Input: part model. Units: mm. Frame: model coordinates. A direction names the side the tool comes from. Round coordinates to 2 decimals unless told otherwise and drop trailing zeros. Order: outer loops, then holes, each group sorted by start corner. A loop starts at its lowest first (then second) coordinate and runs counter-clockwise, first axis right, second up. Notation, with made-up numbers: (-7.75, 39) -> (13.25, 39) arc R23 cw to (13.25, 69) -> close; hole circle Ø4 at (65, 22.5). An arc over 180 degrees is marked (long way). Use a Markdown table: item, result.
from build123d import *

# Parameters (mm, degrees)
SKETCH1_R           = 3.175
BOSS_EXTRUDE1_DEPTH = 6.35
FILLET1_R           = 6.35
FILLET2_R           = 12.7
SKETCH2_R           = 4.9625
CUT_EXTRUDE1_DEPTH  = 4.7625
SKETCH5_R           = 1.778
CUT_EXTRUDE3_DEPTH  = 66.013999766
CUT_EXTRUDE15_DEPTH = 66.013999766
SKETCH11_R          = 3.1702
CUT_EXTRUDE16_DEPTH = 3.175
BOSS_EXTRUDE2_START = -6.35
BOSS_EXTRUDE2_DEPTH = 6.35
SKETCH12_W          = 25.4
SKETCH12_H          = 12.7
CUT_EXTRUDE17_DEPTH = 63.747431864
FILLET14_R          = 3.175
CHAMFER4_SIZE       = 0.4
FILLET16_R          = 3.175
FILLET17_R          = 3.175
SKETCH16_R          = 3.375
BOSS_EXTRUDE4_DEPTH = 6.35
SKETCH17_R          = 3.375
CUT_EXTRUDE19_DEPTH = 69.950310788
FILLET19_R          = 6.35
FILLET20_R          = 9.525


with BuildPart() as part:
    # Sketch1 → Boss-Extrude1 (new body)
    with BuildSketch(Plane.XY):
        with BuildLine():
            Line((-19.735202783, 15.926469991), (-23.822191281, 21.144118554))
            ThreePointArc((-23.822191281, 21.144118554), (-23.438788835, 29.420896018), (-15.197028879, 30.272621002))
            Line((-15.197028879, 30.272621002), (-1.135121582, 20.490721215))
            Line((-1.135121582, 20.490721215), (26.988693011, 20.490721215))
            Line((26.988693011, 20.490721215), (42.638100307, 30.272621002))
            ThreePointArc((42.638100307, 30.272621002), (50.879860264, 29.420896018), (51.263262709, 21.144118554))
            Line((51.263262709, 21.144118554), (47.176274212, 15.926469991))
            Line((47.176274212, 15.926469991), (47.176274212, 5.491172866))
            Line((47.176274212, 5.491172866), (51.263262709, 0.273524304))
            ThreePointArc((51.263262709, 0.273524304), (52.267035248, -1.571068231), (52.614285714, -3.642178571))
            Line((52.614285714, -3.642178571), (52.614285714, -37.65945571))
            Line((52.614285714, -37.65945571), (-25.173214286, -37.65945571))
            Line((-25.173214286, -37.65945571), (-25.173214286, -3.642178571))
            ThreePointArc((-25.173214286, -3.642178571), (-24.825963819, -1.571068231), (-23.822191281, 0.273524304))
            Line((-23.822191281, 0.273524304), (-19.735202783, 5.491172866))
            Line((-19.735202783, 5.491172866), (-19.735202783, 15.926469991))
        make_face()
        with Locations((-18.823214286, 25.059821429)):
            Circle(SKETCH1_R, mode=Mode.SUBTRACT)
        with Locations((46.264285714, 25.059821429)):
            Circle(SKETCH1_R, mode=Mode.SUBTRACT)
        with Locations((46.264285714, -3.642178571)):
            Circle(SKETCH1_R, mode=Mode.SUBTRACT)
        with Locations((-18.823214286, -3.642178571)):
            Circle(SKETCH1_R, mode=Mode.SUBTRACT)
    extrude(amount=BOSS_EXTRUDE1_DEPTH)

    # Fillet1
    fillet1_edges = [part.edges().sort_by_distance(p)[0] for p in [
        (47.176274212, 15.926469991, 3.175),
        (47.176274212, 5.491172866, 3.175),
        (-19.735202783, 5.491172866, 3.175),
        (-19.735202783, 15.926469991, 3.175),
    ]]
    fillet(fillet1_edges, radius=FILLET1_R)

    # Fillet2
    fillet2_edges = [part.edges().sort_by_distance(p)[0] for p in [
        (-1.135121582, 20.490721215, 3.175),
        (26.988693011, 20.490721215, 3.175),
    ]]
    fillet(fillet2_edges, radius=FILLET2_R)

    # Sketch2 → Cut-Extrude1 (cut)
    with BuildSketch(Plane.XY.offset(6.35)):
        with Locations((-18.823214286, 25.059821429)):
            Circle(SKETCH2_R)
        with Locations((-18.823214286, -3.642178571)):
            Circle(SKETCH2_R)
        with Locations((46.264285714, -3.642178571)):
            Circle(SKETCH2_R)
        with Locations((46.264285714, 25.059821429)):
            Circle(SKETCH2_R)
    extrude(amount=-CUT_EXTRUDE1_DEPTH, mode=Mode.SUBTRACT)

    # Sketch5 → Cut-Extrude3 (cut, through all)
    with BuildSketch(Plane(origin=(0, 0, 0), x_dir=(-1, 0, 0), z_dir=(0, 0, -1))):
        with Locations((21.423664788, -18.813799362)):
            Circle(SKETCH5_R)
        with Locations((21.423664788, -28.813754296)):
            Circle(SKETCH5_R)
        with Locations(Location((-26.876213212, -28.813754296, 0), (0, 0, 180))):
            Circle(SKETCH5_R)
        with Locations(Location((-26.876213212, -18.813799362, 0), (0, 0, 180))):
            Circle(SKETCH5_R)
    extrude(amount=-CUT_EXTRUDE3_DEPTH, mode=Mode.SUBTRACT)

    # Sketch6 → Cut-Extrude15 (cut, through all)
    with BuildSketch(Plane.XY.offset(6.35)):
        Polygon((-18.228725788, -33.59545571), (-25.173214286, -33.59545571), (-25.173214286, -37.65945571), (-17.553214286, -37.65945571), (-8.028214286, -37.65945571), (33.881785714, -37.65945571), (43.406785714, -37.65945571), (51.026785714, -37.65945571), (52.614285714, -37.65945571), (52.614285714, -4.530802681), (52.3703532, -5.385290691), (44.317137236, -33.59545571), (23.681274212, -33.59545571), (23.681274212, -13.78345571), (-18.228725788, -13.78345571), align=None)
    extrude(amount=-CUT_EXTRUDE15_DEPTH, mode=Mode.SUBTRACT)

    # Sketch11 → Cut-Extrude16 (cut)
    with BuildSketch(Plane.XY.offset(6.35)):
        with Locations((-21.423664788, -18.813799362)):
            Circle(SKETCH11_R)
        with Locations((-21.423664788, -28.813754296)):
            Circle(SKETCH11_R)
        with Locations((26.876213212, -28.813754296)):
            Circle(SKETCH11_R)
        with Locations((26.876213212, -18.813799362)):
            Circle(SKETCH11_R)
    extrude(amount=-CUT_EXTRUDE16_DEPTH, mode=Mode.SUBTRACT)

    # Sketch13 → Boss-Extrude2 (add)
    with BuildSketch(Plane.XY.offset(6.35).offset(BOSS_EXTRUDE2_START)):
        with BuildLine():
            Line((-30.928725788, -33.59545571), (-25.173214286, -33.59545571))
            Line((-25.173214286, -33.59545571), (-25.173214286, -3.642178571))
            ThreePointArc((-25.173214286, -3.642178571), (-24.825963819, -1.571068231), (-23.822191281, 0.273524304))
            Line((-23.822191281, 0.273524304), (-23.804629036, 0.295945121))
            Line((-23.804629036, 0.295945121), (-30.928725788, -8.632865637))
            Line((-30.928725788, -8.632865637), (-30.928725788, -33.59545571))
        make_face()
    extrude(amount=BOSS_EXTRUDE2_DEPTH)

    # Sketch12 → Cut-Extrude17 (cut, through all)
    with BuildSketch(Plane.XY.offset(6.35)):
        with Locations((12.7, 4.358821429)):
            Rectangle(SKETCH12_W, SKETCH12_H)
    extrude(amount=-CUT_EXTRUDE17_DEPTH, mode=Mode.SUBTRACT)

    # Fillet14
    fillet14_edges = [part.edges().sort_by_distance(p)[0] for p in [
        (0, -1.991178571, 3.175),
        (0, 10.708821429, 3.175),
        (25.4, 10.708821429, 3.175),
        (25.4, -1.991178571, 3.175),
    ]]
    fillet(fillet14_edges, radius=FILLET14_R)

    # Chamfer4
    chamfer4_edges = [part.edges().sort_by_distance(p)[0] for p in [
        (12.7, 10.708821429, 6.35),
        (12.7, 10.708821429, 0),
        (25.4, 4.358821429, 6.35),
        (25.4, 4.358821429, 0),
        (0, 4.358821429, 6.35),
        (0, 4.358821429, 0),
        (12.7, -1.991178571, 6.35),
        (12.7, -1.991178571, 0),
        (24.47006403, 9.778885459, 6.35),
        (24.47006403, 9.778885459, 0),
        (0.92993597, 9.778885459, 6.35),
        (0.92993597, 9.778885459, 0),
        (0.92993597, -1.061242602, 6.35),
        (0.92993597, -1.061242602, 0),
        (24.47006403, -1.061242602, 6.35),
        (24.47006403, -1.061242602, 0),
    ]]
    chamfer(chamfer4_edges, length=CHAMFER4_SIZE)

    # Fillet16
    fillet16_edges = [part.edges().sort_by_distance(p)[0] for p in [
        (-30.928725788, -33.59545571, 3.175),
        (-30.928725788, -8.632865637, 3.175),
    ]]
    fillet(fillet16_edges, radius=FILLET16_R)

    # Fillet17
    fillet17_edges = [part.edges().sort_by_distance(p)[0] for p in [
        (44.317137236, -33.59545571, 3.175),
    ]]
    fillet(fillet17_edges, radius=FILLET17_R)

    # Sketch16 → Boss-Extrude4 (add)
    # profile 1 of 2: a face of its own
    with BuildSketch(Plane.XY.offset(6.35)):
        with BuildLine():
            Line((53.526274212, -9.864372385), (51.091700197, -9.864372385))
            Line((51.091700197, -9.864372385), (50.933736593, -10.417713977))
            ThreePointArc((50.933736593, -10.417713977), (47.420206722, -14.471260278), (48.26426853, -19.768777567))
            Line((48.26426853, -19.768777567), (47.466204116, -22.564372385))
            Line((47.466204116, -22.564372385), (53.526274212, -22.564372385))
            ThreePointArc((53.526274212, -22.564372385), (59.876274212, -16.214372385), (53.526274212, -9.864372385))
        make_face()
        with Locations((53.526274212, -16.214372385)):
            Circle(SKETCH16_R, mode=Mode.SUBTRACT)
    # profile 2 of 2: a face of its own
    with BuildSketch(Plane.XY.offset(6.35)):
        with BuildLine():
            ThreePointArc((-22.681328216, -15.903739098), (-35.032010869, -14.159375941), (-24.200053563, -20.344104369))
            ThreePointArc((-24.200053563, -20.344104369), (-24.423265633, -17.787854523), (-22.681328216, -15.903739098))
        make_face()
        with Locations((-29.023725788, -16.214372385)):
            Circle(SKETCH16_R, mode=Mode.SUBTRACT)
    extrude(amount=-BOSS_EXTRUDE4_DEPTH)

    # Sketch17 → Cut-Extrude19 (cut, through all)
    with BuildSketch(Plane.XY.offset(6.35)):
        with Locations((-29.023725788, -16.214372385)):
            Circle(SKETCH17_R)
    extrude(amount=-CUT_EXTRUDE19_DEPTH, mode=Mode.SUBTRACT)

    # Fillet19
    fillet19_edges = [part.edges().sort_by_distance(p)[0] for p in [
        (-30.928725788, -10.156858456, 3.175),
    ]]
    fillet(fillet19_edges, radius=FILLET19_R)

    # Fillet20
    # the kernel refuses this fillet: 9.525 mm, written as the material it adds along each edge
    with BuildSketch(Plane(origin=(47.466204116, -22.564372385, 6.35), x_dir=(-0.2745058436063301, -0.9615854313715329, 0), z_dir=(0, 0, -1))) as fillet20_piece_1:
        with BuildLine():
            CenterArc((7.143922461, -9.525), FILLET20_R, 90, 69.956718792)
            Line((-1.804186302, -6.260497806), (-2.698997178, -5.934047587))
            ThreePointArc((-2.698997178, -5.934047587), (-2.579434777, -5.565808302), (-0.915910123, 0.261466816))
            Line((-0.915910123, 0.261466816), (0, 0.9525))
            Line((0, 0.9525), (7.143922461, 0.9525))
            Line((7.143922461, 0.9525), (7.143922461, 0))
        make_face()
    extrude(amount=6.35)
    with BuildSketch(Plane(origin=(51.091700197, -9.864372385, 6.35), x_dir=(0.9862513766941969, -0.1652519953549774, 0), z_dir=(0, 0, -1))) as fillet20_piece_2:
        with BuildLine():
            CenterArc((9.56317932, -8.790567042), FILLET20_R, 112.647072848, 47.218605044)
            Line((0.620269026, -5.511850758), (-0.274022003, -5.18397913))
            ThreePointArc((-0.274022003, -5.18397913), (-0.63639102, -2.862441411), (-0.946525533, -0.106516032))
            Line((-0.946525533, -0.106516032), (0.157402526, 0.939404436))
            ThreePointArc((0.157402526, 0.939404436), (2.558504499, 0.537086223), (5.528779384, 0.879056704))
            Line((5.528779384, 0.879056704), (5.895543014, 0))
        make_face()
    extrude(amount=6.35)
    with BuildSketch(Plane(origin=(-30.928725788, -22.271886314, 0), x_dir=(-0.8502967315537753, 0.5263035894889632, 0), z_dir=(0, 0, 1))) as fillet20_piece_3:
        with BuildLine():
            CenterArc((5.488966177, 9.22993895), FILLET20_R, 211.756041781, 43.945519562)
            Line((-2.610110191, 4.21689726), (-2.772091718, 4.116636426))
            Line((-2.772091718, 4.116636426), (-0.161981527, -0.100260834))
            Line((-0.161981527, -0.100260834), (0.047048282, -0.184598779))
            ThreePointArc((0.047048282, -0.184598779), (1.568276051, 0.006207367), (3.08950382, -0.184598779))
            Line((3.08950382, -0.184598779), (3.136552101, 0))
        make_face()
    extrude(amount=6.35)


solid = part.part
1) Pull-direction query (Y, two-part tool) for faces 4 (the flat face through (-18.229, -24, 3)), 5 (the cylindrical face through (29.9, -27.86, 4.78)), 6 (the cylindrical face through (59.66, -17.86, 3.22)), 7 (the cylindrical face through (43.092, 25.199, 0.783)); classes: +Y half, -Y half, draft (parallel to the pull), parting line (faces both ways), or undercut.
Results found:
| item | result |
|---|---|
| face 4 | draft |
| face 5 | undercut |
| face 6 | parting line |
| face 7 | undercut |
2) Line query: L1, parallel to X at y = 22.5, z = 3; L2, parallel to Y at x = 16, z = 4.25; L3, parallel to Y at x = -17, z = 2. Output: solid intervals per line, ascending. Write a range as [from, to].
Results found:
| item | result |
|---|---|
| L1 | x = [-24.63, -23.07], [-14.57, -4.01], [30.2, 42.01], [50.52, 52.08] |
| L2 | y = [-13.78, -1.99], [10.71, 20.49] |
| L3 | y = [-13.78, -8.26], [0.97, 20.44], [29.68, 31.14] |
3) Set-up query: faces 1 (the cylindrical face through (-19.47, 29.98, 4)), 2 (the flat face through (-19.735, 11, 3)), 3 (the cylindrical face through (47.53, 15.83, 3.22)). Return all of +Z, -Z, +X, -X, +Y, -Y with unobstructed straight access to the full face (end or side cutting, diameter ignored); none if empty.
Results found:
| item | result |
|---|---|
| face 1 | +Z |
| face 2 | +Z, -Z, -X |
| face 3 | +Z, -Z, +X |
4) Cut plane B-B on x = 27. Return loops of the section in (y, z) (3 decimals).
Results found:
| item | result |
|---|---|
| outline | (-33.595, 0) -> (-30.587, 0) -> (-30.587, 3.175) -> (-31.982, 3.175) -> (-31.982, 6.35) -> (-33.595, 6.35) -> close; (-27.04, 0) -> (-20.587, 0) -> (-20.587, 3.175) -> (-21.982, 3.175) -> (-21.982, 6.35) -> (-25.646, 6.35) -> (-25.646, 3.175) -> (-27.04, 3.175) -> close; (-17.04, 0) -> (21.028, 0) -> (21.028, 6.35) -> (-15.646, 6.35) -> (-15.646, 3.175) -> (-17.04, 3.175) -> close |
5) Pin query (flat end, axial travel): pin 1 Ø4.5 at (x, y) = (26.88, -18.81) entering from +Z (3 decimals); pin 2 Ø3 at (x, y) = (-16.5, 26) entering from +Z; pin 3 Ø5.5 at (x, y) = (53.53, -16.21) entering from +Z; pin 4 Ø1.9 at (x, z) = (8.5, 4) entering from +Y. Return the tip coordinate at first contact, or that it passes through.
Results found:
| item | result |
|---|---|
| pin 1 | stops at z = 3.175 |
| pin 2 | stops at z = 1.59 |
| pin 3 | passes through |
| pin 4 | stops at y = 20.49 |
6) Cut plane A-A on x = 9.5. Return loops of the section in (y, z), and give its area (3 significant figures).
Results found:
| item | result |
|---|---|
| outline | (-13.78, 0) -> (-2.39, 0) -> (-1.99, 0.4) -> (-1.99, 5.95) -> (-2.39, 6.35) -> (-13.78, 6.35) -> close; (10.71, 0.4) -> (11.11, 0) -> (20.49, 0) -> (20.49, 6.35) -> (11.11, 6.35) -> (10.71, 5.95) -> close |
| area | 137 mm² |
7) Cut plane C-C on x = -10.5. Return loops of the section in (y, z), and give its area (3 significant figures).
Results found:
| item | result |
|---|---|
| outline | (-13.78, 0) -> (27.01, 0) -> (27.01, 6.35) -> (-13.78, 6.35) -> close |
| area | 259 mm² |
